The listing builds one solid part. Answer for the finished solid, in the listing's coordinates (mm). A direction names the side the tool comes from. Coordinates: 2 decimals unless noted, no trailing zeros. Write each loop counter-clockwise with the first axis right and the second up, starting at its lowest first coordinate (ties: lowest second). Pieces come first, ordered by that corner, then holes.
(1) Straight lines are drawn through the part: line 1 (Y direction, x = -0.5, z = 25); line 2 (Z direction, x = 9, y = -30.5); line 3 (Y direction, x = 8, z = 42). For each, find the intervals that lie inside material, in ascending order.
(2) The part is cut by section B-B on z = 34.5. Determine the outline of the cut face in (x, y), plus the area to 3 significant figures.
(3) For a pull along Y with two mould halves and no side action, classify faces 5 (the flat face through (0, 41, 60)), 6 (the flat face through (-26, 0, 60)), 7 (the cylindrical face through (0, 20, 27)) as +Y half, -Y half, draft (parallel to the pull), parting line (faces both ways), or undercut.
(4) Given P1, Ø17, axis at x = -19.5, z = 31, coming from the -Y side; P2, Ø11, axis at x = 20, y = 26, coming from the -Z side; P3, Ø1.5, axis at y = 17, z = 8, coming from the -X side, each flat-ended and moving along its own axis, determine where each tip first touches the part or whether it passes through.
(5) Which of the six approach directions +Z, -Z, +X, -X, +Y, -Y give full straight-line access (tool end or side, diameter ignored) to faces 1 (the cylindrical face through (0, -20, 27)), 2 (the flat face through (17, -10, 42)), 3 (the flat face through (-1, 28, 55)), 4 (the flat face through (-17, 10, 37))?
(6) The part is cut by section D-D on y = -36.5. Determine the outline of the cut face in (x, z).
(7) The part is cut by section A-A on x = 0. Determine the outline of the cut face in (y, z), plus the area to 3 significant figures.
(8) The part is cut by section C-C on y = 12. Determine the outline of the cut face in (x, z), plus the area to 3 significant figures.
Autodesk Fusion 360 part; units mm, degrees
sketch "スケッチ1" plane through (0, 0, 0) normal (0, 0, 1) x (1, 0, 0)
  circle A0 centre (0, 0) radius 46
  dimension "d1" = 92
extrude "押し出し1" add sketch "スケッチ1" along normal blind 70
sketch "スケッチ2" plane through (0, 0, 70) normal (0, 0, 1) x (-1, 0, 0)
  circle A0 centre (0, 0) radius 46
  circle A1 centre (0, 0) radius 40.5
  dimension "d4" = 81
extrude "押し出し2" cut sketch "スケッチ2" against normal blind 10
sketch "スケッチ3" plane through (0, 0, 70) normal (0, 0, 1) x (-1, 0, 0)
  circle A0 centre (0, 0) radius 40.5
  circle A1 centre (0, 0) radius 15
  dimension "d7" = 30
extrude "押し出し3" cut sketch "スケッチ3" against normal blind 100 contours A1
sketch "スケッチ4" plane through (0, 0, 0) normal (0, 0, -1) x (1, 0, 0)
  circle A0 centre (0, 0) radius 15
  circle A1 centre (0, 0) radius 46
  circle A2 centre (0, 0) radius 20
  dimension "d12" = 40
extrude "押し出し4" cut sketch "スケッチ4" against normal blind 55 contours A1
sketch "スケッチ5" plane through (0, 0, 0) normal (0, 0, -1) x (1, 0, 0)
  circle A0 centre (0, 0) radius 20
  circle A1 centre (0, 0) radius 15
  line L0 (-55, 10) -> (55, 10)
  line L1 (55, 10) -> (55, -10)
  line L2 (55, -10) -> (-55, -10)
  line L3 (-55, -10) -> (-55, 10)
extrude "押し出し5" cut sketch "スケッチ5" against normal blind 60 contours A0 A1 L0 L2 | A0 L0 L1 L2 | A0 A1 L0 L2 | A0 L0 L2 L3
extrude "押し出し6" cut 1 faces at (31.4239, 5.7402, 60) along direction (0, 0, 1) blind 10
fillet "フィレット1" [suppressed]
Model answer:
1. line 1: y = -19.99 to -14.99, 14.99 to 19.99
1. line 2: z = 55 to 70
1. line 3: y = -18.33 to -12.69, 12.69 to 18.33
2. outline: (-17.32, -10) arc R20 ccw to (17.32, -10) - (11.18, -10) arc R15 cw to (-11.18, -10) - close; (-17.32, 10) - (-11.18, 10) arc R15 cw to (11.18, 10) - (17.32, 10) arc R20 ccw to start
2. area: 336 mm2
3. face 5: draft
3. face 6: undercut
3. face 7: +Y half
4. P1: stops at y = -16.7
4. P2: stops at z = 55
4. P3: stops at x = -11.66
5. face 1: -Z, -Y
5. face 2: +Z, -Z, +X
5. face 3: -Z, +Y
5. face 4: -Z, +X, -X
6. outline: (-28, 55) - (28, 55) - (28, 60) - (17.55, 60) - (17.55, 70) - (-17.55, 70) - (-17.55, 60) - (-28, 60) - close
7. outline: (-46, 55) - (-20, 55) - (-20, 0) - (-15, 0) - (-15, 70) - (-40.5, 70) - (-40.5, 60) - (-46, 60) - close; (15, 0) - (20, 0) - (20, 55) - (46, 55) - (46, 60) - (40.5, 60) - (40.5, 70) - (15, 70) - close
7. area: 1,370 mm2
8. outline: (-44.41, 55) - (-16, 55) - (-16, 0) - (-9, 0) - (-9, 70) - (-38.68, 70) - (-38.68, 60) - (-44.41, 60) - close; (9, 0) - (16, 0) - (16, 55) - (44.41, 55) - (44.41, 60) - (38.68, 60) - (38.68, 70) - (9, 70) - close
8. area: 1,720 mm2
